from build123d import *

# Parameters (mm, degrees)
SKETCH1_W                             = 16
SKETCH1_H                             = 16
SHAFT_SUPPORT_DEPTH                   = 38
D8_GUIDE_SHAFT_SEAT_DEPTH             = 40.648455203
D8_GUIDE_SHAFT_SEAT_DEPTH_BACK        = 40.648455203
SKETCH2_R                             = 4
SKETCH3_R                             = 2.5
M5_BOTTOM_THREAD_MAJOR_ENVELOPE_DEPTH = 8


with BuildPart() as part:
    # Sketch1 → Shaft_Support (new body)
    with BuildSketch(Plane.XY):
        Rectangle(SKETCH1_W, SKETCH1_H)
    extrude(amount=SHAFT_SUPPORT_DEPTH)

    # Sketch2 → D8_Guide_Shaft_Seat (cut, two sides: drawn at the far end of the back side and taken through both)
    with BuildSketch(Plane(origin=(0, 0, 0), x_dir=(1, 0, 0), z_dir=(0, 1, 0)).offset(-D8_GUIDE_SHAFT_SEAT_DEPTH_BACK)):
        with Locations(Location((0, -30, 0), (0, 0, 270))):
            Circle(SKETCH2_R)
    extrude(amount=D8_GUIDE_SHAFT_SEAT_DEPTH + D8_GUIDE_SHAFT_SEAT_DEPTH_BACK, mode=Mode.SUBTRACT)

    # Sketch3 → M5_Bottom_Thread_Major_Envelope (cut)
    with BuildSketch(Plane(origin=(0, 0, 0), x_dir=(-1, 0, 0), z_dir=(0, 0, -1))):
        Circle(SKETCH3_R)
    extrude(amount=-M5_BOTTOM_THREAD_MAJOR_ENVELOPE_DEPTH, mode=Mode.SUBTRACT)


solid = part.part
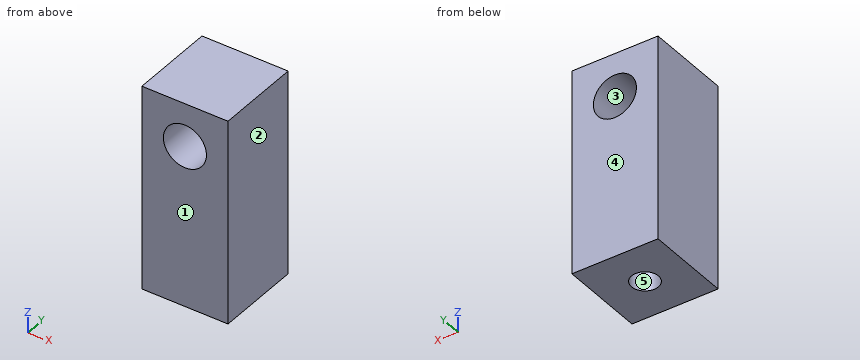
Check sheet for the modelled part. Datum: model origin and axes. Units: mm. Face numbers are marked on the shaded views. A direction names the side the tool comes from. Give positions to 0.01 mm unless a question says otherwise; leave off trailing zeros. Loops run counter-clockwise (first coordinate to the right, second up) from the corner with the lowest first, then second, coordinate; pieces in that order, holes last. Notation, with made-up numbers: M -1.75,-12.75 L 27.25,-12.75 A30 ccw 27.25,14.25 Z; hole C 14,-7 d7. An arc over 180 degrees is marked long. Return JSON: item names as keys, results as strings. Group by question number.
1. Thickness scan on L1, parallel to Y at x = 0, z = 2.5; L2, parallel to X at y = -1, z = 30; L3, parallel to Z at x = 0, y = -1. Record the ranges inside material, lowest first.
2. Tool access check on the marked faces 4 and 5. Record the directions out of +Z, -Z, +X, -X, +Y, -Y that give a thin tool (end or side, any length) a straight path to the whole face; none if there is none.
3. Cross-section at A-A on z = 30. Record the boundary of the cut face in (x, y), plus the area to 3 significant figures.
4. Mould release check, pull along X, two halves, no side actions. Record for the marked faces 1, 2 and 3: released by +X, released by -X, zero draft, split by the parting line, or undercut.
5. Cross-section at D-D on z = 6.5. Record the boundary of the cut face in (x, y).
6. Cross-section at C-C on x = 0. Record the boundary of the cut face in (y, z).
7. Cross-section at B-B on y = 0. Record the boundary of the cut face in (x, z).
Return value:
{
 "1": {"L1": "-8 to -2.5, 2.5 to 8", "L2": "-8 to -4, 4 to 8", "L3": "8 to 26, 34 to 38"},
 "2": {"face 4": "+Z, -Z, +X, -X, +Y", "face 5": "-Z"},
 "3": {"outline": "M -8,-8 L -4,-8 L -4,8 L -8,8 Z; M 4,-8 L 8,-8 L 8,8 L 4,8 Z", "area": "128 mm^2"},
 "4": {"face 1": "zero draft", "face 2": "released by +X", "face 3": "undercut"},
 "5": {"outline": "M -8,-8 L 8,-8 L 8,8 L -8,8 Z; hole C 0,0 d5"},
 "6": {"outline": "M -8,0 L -2.5,0 L -2.5,8 L 2.5,8 L 2.5,0 L 8,0 L 8,26 L -8,26 Z; M -8,34 L 8,34 L 8,38 L -8,38 Z"},
 "7": {"outline": "M -8,0 L -2.5,0 L -2.5,8 L 2.5,8 L 2.5,0 L 8,0 L 8,38 L -8,38 Z; hole C 0,30 d8"}
}
